Here's how the part is built. I have some questions about the finished solid (model axes, mm). A direction names the side the tool comes from. Coordinates: 2 decimals unless noted, no trailing zeros. Loops run counter-clockwise (first coordinate to the right, second up) from the corner with the lowest first, then second, coordinate; pieces in that order, holes last. Notation, with made-up numbers: M -21,73 L 29,73 A22 cw 29,84 Z; hole C 79.5,41 d7. An arc over 180 degrees is marked long. Use one line per item in the form item = value. Start each with the question number.
(1) Please list where these lines run through material, in increasing order: L1, parallel to X at y = 91, z = 0; L2, parallel to Z at x = 0, y = 3.65; L3, parallel to Z at x = 13.5, y = 5.
(2) Will these pins go through, and if not, where does the flat tip stop? P1, Ø4.5, axis at x = 12.12, z = 7, coming from the -Y side; P2, Ø12, axis at y = 75.5, z = -11, coming from the +X side; P3, Ø3.5, axis at x = 0, z = 14, coming from the -Y side; P4, Ø4, axis at y = 14, z = -0.5, coming from the -X side.
(3) Imagine slicing it at B-B, the plane y = 91. Please give me the cut outline in (x, z).
(4) Imagine slicing it at A-A, the plane x = 0. Please give me the cut outline in (y, z), and give its area (3 significant figures).
(5) Imagine slicing it at D-D, the plane z = -14. Please give me the cut outline in (x, y), and give its area (3 significant figures).
(6) On a 3-axis mill with a long thin cutter (end or side, diameter ignored), from which of +Z, -Z, +X, -X, +Y, -Y can I reach the whole of each face in a straight line? I mean faces 1 (the cylindrical face through (0, 3, -16)), 2 (the flat face through (8, 6, 0)). Say none if no direction works.
(7) Imagine slicing it at C-C, the plane x = 12. Please give me the cut outline in (y, z), and give its area (3 significant figures).
(8) Thinking about a two-plate mould opening in Y: for faces 3 (the flat face through (0, 96, 0)), 4 (the cylindrical face through (14.032, 3.042, 6.399)), 5 (the cylindrical face through (1.666, 89.722, -0.101)), which applies, +Y half, -Y half, draft (parallel to the pull), parting line (faces both ways), or undercut?
```python
from build123d import *

# Parameters (mm, degrees)
SKETCH1_R           = 18.2
BOSS_EXTRUDE1_DEPTH = 6
SKETCH3_R           = 2
CUT_EXTRUDE1_DEPTH  = 10
CIRPATTERN1_COUNT   = 6
SKETCH4_R           = 7.5
BOSS_EXTRUDE2_DEPTH = 90
SKETCH9_R           = 2.1
CUT_EXTRUDE2_DEPTH  = 26.7


with BuildPart() as part:
    # Sketch1 → Boss-Extrude1 (new body)
    with BuildSketch(Plane(origin=(0, 0, 0), x_dir=(1, 0, 0), z_dir=(0, 1, 0))):
        Circle(SKETCH1_R)
    extrude(amount=BOSS_EXTRUDE1_DEPTH)

    # Sketch3 → Cut-Extrude1 (cut)
    with BuildSketch(Plane(origin=(0, 6, 0), x_dir=(1, 0, 0), z_dir=(0, 1, 0))):
        with Locations((0, 14)):
            Circle(SKETCH3_R)
    cut_extrude1 = extrude(amount=-CUT_EXTRUDE1_DEPTH, mode=Mode.SUBTRACT)

    # CirPattern1: Cut-Extrude1 ×6 about axis
    cirpattern1_axis = Axis((0, 0, 0), (0, 1, 0))
    for i in range(1, CIRPATTERN1_COUNT):
        add(cut_extrude1.rotate(cirpattern1_axis, i * 360 / CIRPATTERN1_COUNT), mode=Mode.SUBTRACT)

    # Sketch4 → Boss-Extrude2 (add)
    with BuildSketch(Plane(origin=(0, 6, 0), x_dir=(1, 0, 0), z_dir=(0, 1, 0))):
        Circle(SKETCH4_R)
    extrude(amount=BOSS_EXTRUDE2_DEPTH)

    # Sketch9 → Cut-Extrude2 (cut, through all)
    with BuildSketch(Plane(origin=(0, 0, -7.5), x_dir=(-1, 0, 0), z_dir=(0, 0, -1))):
        with Locations((0, 91)):
            Circle(SKETCH9_R)
    extrude(amount=-CUT_EXTRUDE2_DEPTH, mode=Mode.SUBTRACT)


solid = part.part
```
Answer:
q1.L1 = -7.5 to -2.1, 2.1 to 7.5
q1.L2 = -18.2 to -16, -12 to 12, 16 to 18.2
q1.L3 = -12.21 to -8.45, -5.55 to 5.55, 8.45 to 12.21
q2.P1 = 0
q2.P2 = 5.59
q2.P3 = through
q2.P4 = -7.5
q3.outline = M -2.1,-7.2 L -2.1,7.2 A7.5 ccw Z; M 2.1,-7.2 A7.5 ccw 2.1,7.2 Z
q4.outline = M 0,-18.2 L 6,-18.2 L 6,-16 L 0,-16 Z; M 0,-12 L 6,-12 L 6,-7.5 L 88.9,-7.5 L 88.9,7.5 L 6,7.5 L 6,12 L 0,12 Z; M 0,16 L 6,16 L 6,18.2 L 0,18.2 Z; M 93.1,-7.5 L 96,-7.5 L 96,7.5 L 93.1,7.5 Z
q4.area = 1,460 mm²
q5.outline = M -11.63,0 L -2,0 L -2,6 L -11.63,6 Z; M 2,0 L 11.63,0 L 11.63,6 L 2,6 Z
q5.area = 116 mm²
q6.face_1 = +Y, -Y
q6.face_2 = +Y
q7.outline = M 0,-13.68 L 6,-13.68 L 6,-9 L 0,-9 Z; M 0,-5 L 6,-5 L 6,5 L 0,5 Z; M 0,9 L 6,9 L 6,13.68 L 0,13.68 Z
q7.area = 116 mm²
q8.face_3 = +Y half
q8.face_4 = draft
q8.face_5 = undercut
